```python
from build123d import *

# Parameters (mm, degrees)
F0_R     = 1.541714
F1_DEPTH = 5.25


with BuildPart() as f1:
    # F0 (on Top) → F1 (new body)
    with BuildSketch(Plane.XY):
        with BuildLine():
            add(Edge.make_bspline(
                [(-39.234068, 14.709434), (-35.821676, 18.285589), (-31.741335, 20.813416), (-28.060412, 21.400427)],
                knots=[0, 0, 0, 0, 13.023824, 13.023824, 13.023824, 13.023824], degree=3))
            add(Edge.make_bspline(
                [(-39.234068, 14.709434), (-44.434033, 9.709523), (-49.091313, 1.579042), (-48.498575, -7.294206)],
                knots=[0, 0, 0, 0, 23.87449, 23.87449, 23.87449, 23.87449], degree=3))
            add(Edge.make_bspline(
                [(-48.498575, -7.294206), (-48.312098, -9.073281), (-47.466565, -11.387973), (-46.594005, -13.059257)],
                knots=[0, 0, 0, 0, 6.071506, 6.071506, 6.071506, 6.071506], degree=3))
            add(Edge.make_bspline(
                [(-46.594005, -13.059257), (-51.85584, -16.912187), (-55.326007, -21.131784), (-54.675397, -25.848711)],
                knots=[0, 0, 0, 0, 15.128748, 15.128748, 15.128748, 15.128748], degree=3))
            ThreePointArc((-54.675397, -25.848711), (-53.725936, -27.271081), (-52.113619, -27.841207))
            add(Edge.make_bspline(
                [(-52.113619, -27.841207), (-48.665918, -27.506378), (-50.121121, -21.213111), (-43.411698, -16.496183)],
                knots=[0, 0, 0, 0, 14.298006, 14.298006, 14.298006, 14.298006], degree=3))
            ThreePointArc((-43.411698, -16.496183), (-39.541163, -19.502637), (-35.015989, -21.384818))
            add(Edge.make_bspline(
                [(-35.015989, -21.384818), (-37.141673, -30.065609), (-38.5387, -34.983439), (-37.43797, -40.036903)],
                knots=[0, 0, 0, 0, 18.808675, 18.808675, 18.808675, 18.808675], degree=3))
            add(Edge.make_bspline(
                [(-9.984496, -40.036903), (-20.42749, -51.944654), (-36.633965, -45.385001), (-37.43797, -40.036903)],
                knots=[0, 0, 0, 0, 27.453474, 27.453474, 27.453474, 27.453474], degree=3))
            add(Edge.make_bspline(
                [(-9.984496, -14.392133), (1.210287, -24.002717), (-6.147497, -34.946361), (-9.984496, -40.036903)],
                knots=[0, 0, 0, 0, 25.64477, 25.64477, 25.64477, 25.64477], degree=3))
            add(Edge.make_bspline(
                [(-6.307024, 3.602734), (-2.207622, -1.597791), (-7.333158, -11.79279), (-9.984496, -14.392133)],
                knots=[0, 0, 0, 0, 18.326618, 18.326618, 18.326618, 18.326618], degree=3))
            add(Edge.make_bspline(
                [(-31.371076, -8.189144), (-22.531703, 9.364952), (-9.091812, 7.34916), (-6.307024, 3.602734)],
                knots=[0, 0, 0, 0, 27.699369, 27.699369, 27.699369, 27.699369], degree=3))
            add(Edge.make_bspline(
                [(-42.004138, -11.402097), (-36.800269, -9.169074), (-34.760952, -8.423049), (-31.371076, -8.189144)],
                knots=[0, 0, 0, 0, 11.107884, 11.107884, 11.107884, 11.107884], degree=3))
            add(Edge.make_bspline(
                [(-25.930956, 18.182661), (-41.983377, 13.510846), (-46.004765, -6.258437), (-42.004138, -11.402097)],
                knots=[0, 0, 0, 0, 33.669052, 33.669052, 33.669052, 33.669052], degree=3))
            add(Edge.make_bspline(
                [(-19.430624, 14.216358), (-20.169115, 17.171623), (-20.674834, 19.440178), (-25.930956, 18.182661)],
                knots=[0, 0, 0, 0, 7.614846, 7.614846, 7.614846, 7.614846], degree=3))
            add(Edge.make_bspline(
                [(-13.350238, 14.216358), (-12.521998, 11.102053), (-19.320449, 12.233206), (-19.430624, 14.216358)],
                knots=[0, 0, 0, 0, 6.080386, 6.080386, 6.080386, 6.080386], degree=3))
            add(Edge.make_bspline(
                [(-24.679011, 21.678406), (-22.74786, 21.887188), (-14.866098, 22.765726), (-13.350238, 14.216358)],
                knots=[0, 0, 0, 0, 13.565518, 13.565518, 13.565518, 13.565518], degree=3))
            ThreePointArc((-24.679011, 21.678406), (-26.97945, 28.956423), (-28.060412, 21.400427))
        make_face()
        with BuildLine():
            add(Edge.make_bspline(
                [(-40.052891, -14.35038), (-38.893204, -15.726322), (-36.317203, -17.658971), (-34.448564, -17.57047)],
                knots=[0, 0, 0, 0, 6.463548, 6.463548, 6.463548, 6.463548], degree=3))
            add(Edge.make_bspline(
                [(-40.052891, -14.35038), (-38.873214, -13.307477), (-34.543491, -12.330866), (-32.659906, -12.174509)],
                knots=[0, 0, 0, 0, 7.706532, 7.706532, 7.706532, 7.706532], degree=3))
            ThreePointArc((-32.659906, -12.174509), (-33.308264, -14.954024), (-34.448564, -17.57047))
        make_face(mode=Mode.SUBTRACT)
        with BuildLine():
            add(Edge.make_bspline(
                [(-29.753655, -39.981414), (-34.422584, -37.67078), (-31.337596, -28.266594), (-29.212372, -21.832947)],
                knots=[0, 0, 0, 0, 18.156537, 18.156537, 18.156537, 18.156537], degree=3))
            add(Edge.make_bspline(
                [(-29.212372, -21.832947), (-22.684187, -21.978017), (-18.670561, -19.801956), (-13.061159, -16.803825)],
                knots=[0, 0, 0, 0, 16.91608, 16.91608, 16.91608, 16.91608], degree=3))
            add(Edge.make_bspline(
                [(-29.753655, -39.981414), (-17.026084, -44.860996), (-4.447781, -25.163252), (-13.061159, -16.803825)],
                knots=[0, 0, 0, 0, 28.562913, 28.562913, 28.562913, 28.562913], degree=3))
        make_face(mode=Mode.SUBTRACT)
        with BuildLine():
            ThreePointArc((-16.616, -14.512614), (-22.063718, -17.107114), (-28.06261, -17.756996))
            ThreePointArc((-28.06261, -17.756996), (-27.051078, -14.329094), (-25.590414, -11.067166))
            add(Edge.make_bspline(
                [(-25.590414, -11.067166), (-23.060093, -10.862005), (-17.589131, -12.503293), (-16.616, -14.512614)],
                knots=[0, 0, 0, 0, 9.613076, 9.613076, 9.613076, 9.613076], degree=3))
        make_face(mode=Mode.SUBTRACT)
        with BuildLine():
            add(Edge.make_bspline(
                [(-23.741798, -7.787112), (-20.216195, -8.558338), (-15.917903, -9.419195), (-12.841488, -11.621797)],
                knots=[0, 0, 0, 0, 11.555154, 11.555154, 11.555154, 11.555154], degree=3))
            add(Edge.make_bspline(
                [(-23.741798, -7.787112), (-19.572357, 0.079918), (-13.183153, 4.161766), (-9.049211, 2.69497)],
                knots=[0, 0, 0, 0, 18.04844, 18.04844, 18.04844, 18.04844], degree=3))
            add(Edge.make_bspline(
                [(-9.049211, 2.69497), (-5.512775, 0.57912), (-9.853426, -9.418107), (-12.841488, -11.621797)],
                knots=[0, 0, 0, 0, 14.81051, 14.81051, 14.81051, 14.81051], degree=3))
        make_face(mode=Mode.SUBTRACT)
        with Locations((-26.658739, 25.055223)):
            Circle(F0_R, mode=Mode.SUBTRACT)
    extrude(amount=F1_DEPTH)


solid = f1.part
```
Read the model definition and answer for the solid it produces. Units are mm, in the model's axes. A direction names the side the tool comes from. Coordinates: 2 decimals unless noted, no trailing zeros. Answer in a Markdown table with one row per item.
1. Which of the six approach directions +Z, -Z, +X, -X, +Y, -Y give full straight-line access (tool end or side, diameter ignored) to faces 4 (the face through (-27, -11, 0)), 5 (the face through (-39.6, -19.47, 2.59))?
Conclusion:
| item | result |
|---|---|
| face 4 | -Z, +X, -X, +Y, -Y |
| face 5 | +Z, -Z |
2. Determine the mould class of faces 1 (the face through (-53.745, -27.256, 2.588)), 2 (the face through (-27, -11, 5.25)), 3 (the face through (-27.795, 26.097, 2.588)) for opening direction Y: +Y half, -Y half, draft (parallel to the pull), parting line (faces both ways), or undercut.
Conclusion:
| item | result |
|---|---|
| face 1 | -Y half |
| face 2 | draft |
| face 3 | undercut |
3. Given pin 1 (1.5 mm diameter, centred on y = -19.5, z = 1, fed in from -X); pin 2 (4 mm diameter, centred on x = -26.66, y = 25.06, fed in from +Z); pin 3 (1.5 mm diameter, centred on x = -14, z = 4, fed in from +Y); pin 4 (1 mm diameter, centred on x = -21.5, z = 4.5, fed in from +Y), each flat-ended and moving along its own axis, determine where each tip first touches the part or whether it passes through.
Conclusion:
| item | result |
|---|---|
| pin 1 | stops at x = -53.54 |
| pin 2 | stops at z = 5.25 |
| pin 3 | stops at y = 18.03 |
| pin 4 | stops at y = 21.79 |
4. Straight lines are drawn through the part: line 1 (X direction, y = -26, z = 1.45); line 2 (Y direction, x = -12, z = 1.5); line 3 (X direction, y = 0.5, z = 3.45). For each, find the intervals that lie inside material, in ascending order.
Conclusion:
| item | result |
|---|---|
| line 1 | x = -54.63 to -49.91, -36.15 to -30.54, -10.39 to -4.04 |
| line 2 | y = -42.05 to -30.96, -18.03 to -10.84, 2.89 to 6.11 |
| line 3 | x = -47.72 to -42.54, -25.28 to -17.01, -7.78 to -4.94 |
5. Find section A-A, the plane y = 1.5. Count the separate pieces of the cut face and the enclosed holes in it, then the cut area to 3 significant figures.
Conclusion:
| item | result |
|---|---|
| separate pieces | 3 |
| enclosed holes | 0 |
| area | 87.8 mm² |
